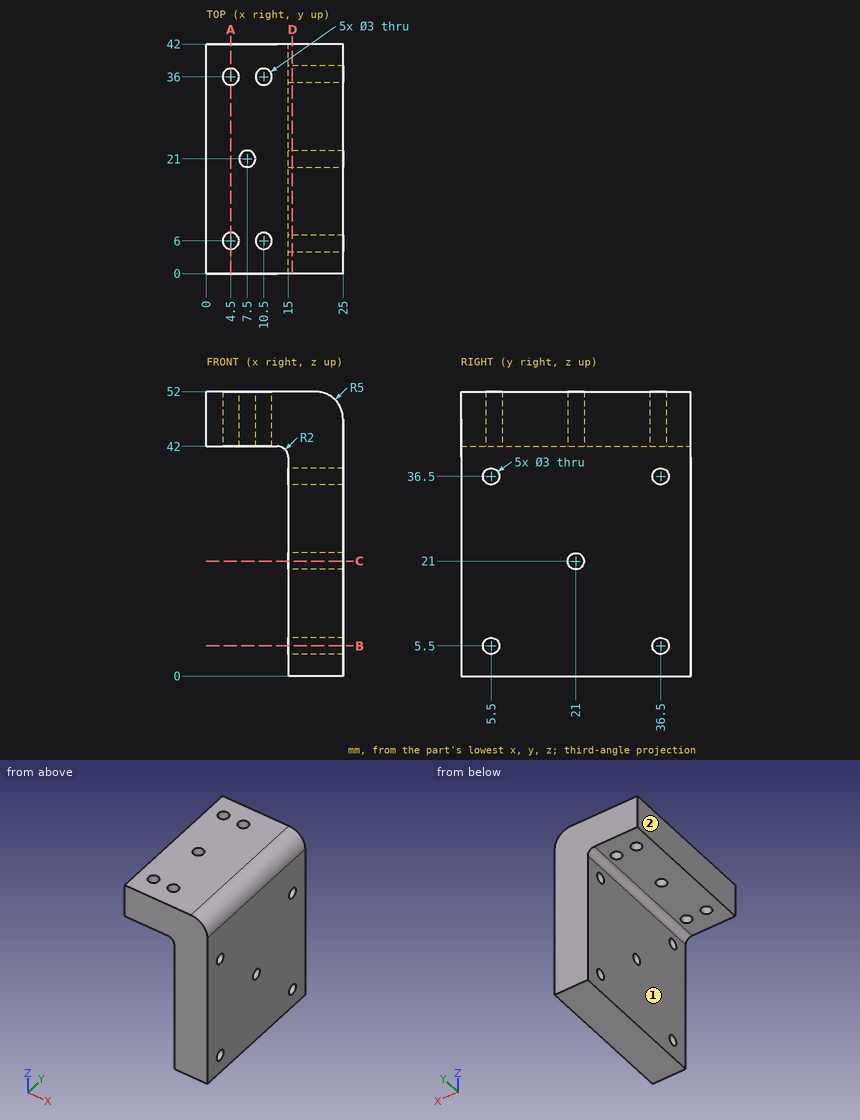
Study the drawing (mm; zero at the part's minimum x, y, z) and answer. A direction names the side the tool comes from. Give positions to 0.01 mm unless a question says otherwise; leave off trailing zeros. Loops run counter-clockwise (first coordinate to the right, second up) from the corner with the lowest first, then second, coordinate; pieces in that order, holes last. Notation, with made-up numbers: (-7, 24) - (10, 24) arc R7 ccw to (10, 34) - close; hole circle Ø1 at (-14.5, 35). An arc over 180 degrees is marked (long way). One line per question, with ' | ' between items.
(1) The part is cut by section D-D (x = 15.75). Write down the section's boundary in (y, z), then the cut area to 3 significant figures.
Recorded:
outline: (0, 0) - (42, 0) - (42, 52) - (0, 52) - close; hole circle Ø3 at (5.5, 5.5); hole circle Ø3 at (5.5, 36.5); hole circle Ø3 at (21, 21); hole circle Ø3 at (36.5, 5.5); hole circle Ø3 at (36.5, 36.5) | area: 2,150 mm²
(2) The part is cut by section C-C (z = 21). Write down the section's boundary in (x, y), then the cut area to 3 significant figures.
Recorded:
outline: (15, 0) - (25, 0) - (25, 19.5) - (15, 19.5) - close; (15, 22.5) - (25, 22.5) - (25, 42) - (15, 42) - close | area: 390 mm²
(3) The part is cut by section A-A (x = 4.5). Write down the section's boundary in (y, z).
Recorded:
outline: (0, 42) - (4.5, 42) - (4.5, 52) - (0, 52) - close; (7.5, 42) - (34.5, 42) - (34.5, 52) - (7.5, 52) - close; (37.5, 42) - (42, 42) - (42, 52) - (37.5, 52) - close
(4) Straight lines are drawn through the part: probe 1 along Y at (x, z) = (10.5, 45.75); probe 2 along Z at (x, y) = (17, 37); probe 3 along X at (y, z) = (30.5, 10). For each, find the intervals that lie inside material, in ascending order.
Recorded:
probe 1: y = 0 to 4.5, 7.5 to 34.5, 37.5 to 42 | probe 2: z = 0 to 4.09, 6.91 to 35.09, 37.91 to 52 | probe 3: x = 15 to 25
(5) Each of these flat-tipped pins is pushed along its axis until it touches: pin 1 Ø5 at (y, z) = (30.5, 13.5) entering from -X; pin 2 Ø2.5 at (y, z) = (36.5, 5.5) entering from +X; pin 3 Ø5 at (x, y) = (10.5, 36) entering from -Z. Where does it stop, or does it pass through?
Recorded:
pin 1: stops at x = 15 | pin 2: passes through | pin 3: stops at z = 42
(6) The part is cut by section B-B (z = 5.5). Write down the section's boundary in (x, y), then the cut area to 3 significant figures.
Recorded:
outline: (15, 0) - (25, 0) - (25, 4) - (15, 4) - close; (15, 7) - (25, 7) - (25, 35) - (15, 35) - close; (15, 38) - (25, 38) - (25, 42) - (15, 42) - close | area: 360 mm²
(7) A tool of negligible diameter and unlimited length cuts with its end or side. For the marked faces 1 and 2, from which of +Z, -Z, +X, -X, +Y, -Y can it reach the whole face along a straight path? Write none if from no direction.
Recorded:
face 1: -Z, -X, +Y, -Y | face 2: +Z, -Z, -X, +Y, -Y
